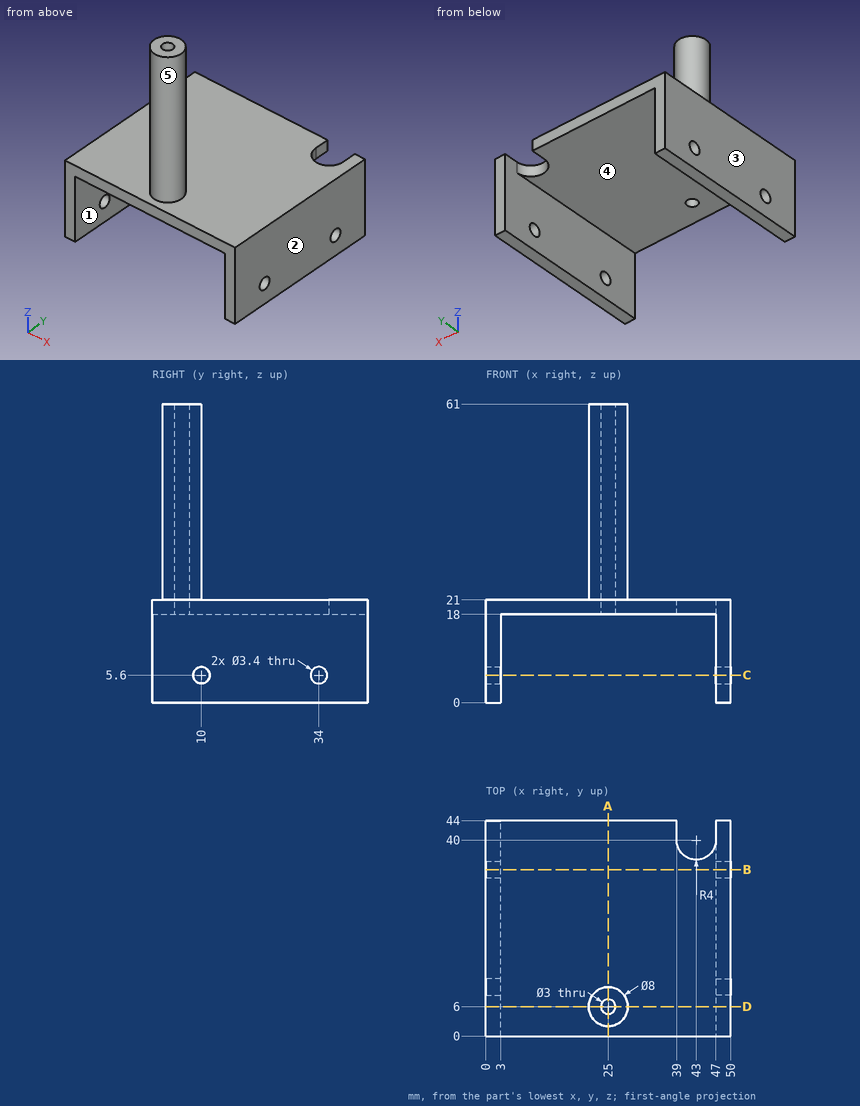
The figure shows three views and two pictorial views of one solid part (mm, origin at its lowest corner). Answer the questions. A direction names the side the tool comes from. Give positions to 0.01 mm unless a question says otherwise; leave off trailing zeros. Write each loop counter-clockwise with the first axis right and the second up, starting at its lowest first coordinate (ties: lowest second). Pieces come first, ordered by that corner, then holes. Notation, with made-up numbers: (62.5, -27) - (69.5, -27) arc R11 ccw to (69.5, -8) - close; hole circle Ø4 at (18, 25). An arc over 180 degrees is marked (long way). Return JSON: item names as keys, results as strings.
Q1. For the marked faces 4 and 5, determine the directions among +Z, -Z, +X, -X, +Y, -Y from which every point of the face is accessible in a straight line to the end or side of a thin tool.
Reply:
{"face 4": "-Z, +Y, -Y", "face 5": "+Z"}
Q2. Consider line 1 along X through (y, z) = (22, 11); line 2 along Z through (x, y) = (48.6, 34); line 3 along Z through (x, y) = (6.5, 34). Determine where each line is inside the solid, lowest interval first. Write a range as [from, to].
Reply:
{"line 1": "[0, 3], [47, 50]", "line 2": "[0, 3.9], [7.3, 21]", "line 3": "[18, 21]"}
Q3. A cutting plane is placed at C-C, the plane z = 5.6. Determine the outline of the cut face in (x, y), and give its area (3 significant figures).
Reply:
{"outline": "(0, 0) - (3, 0) - (3, 8.3) - (0, 8.3) - close; (0, 11.7) - (3, 11.7) - (3, 32.3) - (0, 32.3) - close; (0, 35.7) - (3, 35.7) - (3, 44) - (0, 44) - close; (47, 0) - (50, 0) - (50, 8.3) - (47, 8.3) - close; (47, 11.7) - (50, 11.7) - (50, 32.3) - (47, 32.3) - close; (47, 35.7) - (50, 35.7) - (50, 44) - (47, 44) - close", "area": "223 mm²"}
Q4. A cutting plane is placed at A-A, the plane x = 25. Determine the outline of the cut face in (y, z), and give its area (3 significant figures).
Reply:
{"outline": "(0, 18) - (4.5, 18) - (4.5, 61) - (2, 61) - (2, 21) - (0, 21) - close; (7.5, 18) - (44, 18) - (44, 21) - (10, 21) - (10, 61) - (7.5, 61) - close", "area": "323 mm²"}
Q5. Given P1, Ø1.5, axis at x = 13, z = 21.5, coming from the -Y side; P2, Ø1, axis at x = 44.5, y = 31.5, coming from the -Z side; P3, Ø22, axis at x = 21.5, y = 24.5, coming from the +Z side, each flat-ended and moving along its own axis, determine where each tip first touches the part or whether it passes through.
Reply:
{"P1": "y = 0", "P2": "z = 18", "P3": "z = 21"}
Q6. A cutting plane is placed at D-D, the plane y = 6. Determine the outline of the cut face in (x, z), and give its area (3 significant figures).
Reply:
{"outline": "(0, 0) - (3, 0) - (3, 18) - (23.5, 18) - (23.5, 61) - (21, 61) - (21, 21) - (0, 21) - close; (26.5, 18) - (47, 18) - (47, 0) - (50, 0) - (50, 21) - (29, 21) - (29, 61) - (26.5, 61) - close", "area": "449 mm²"}
Q7. For a pull along X with two mould halves and no side action, classify the marked faces 1, 2 and 3 as released by +X, released by -X, zero draft, split by the parting line, or undercut.
Reply:
{"face 1": "undercut", "face 2": "released by +X", "face 3": "released by -X"}
Q8. A cutting plane is placed at B-B, the plane y = 34. Determine the outline of the cut face in (x, z).
Reply:
{"outline": "(0, 0) - (3, 0) - (3, 3.9) - (0, 3.9) - close; (0, 7.3) - (3, 7.3) - (3, 18) - (47, 18) - (47, 7.3) - (50, 7.3) - (50, 21) - (0, 21) - close; (47, 0) - (50, 0) - (50, 3.9) - (47, 3.9) - close"}
